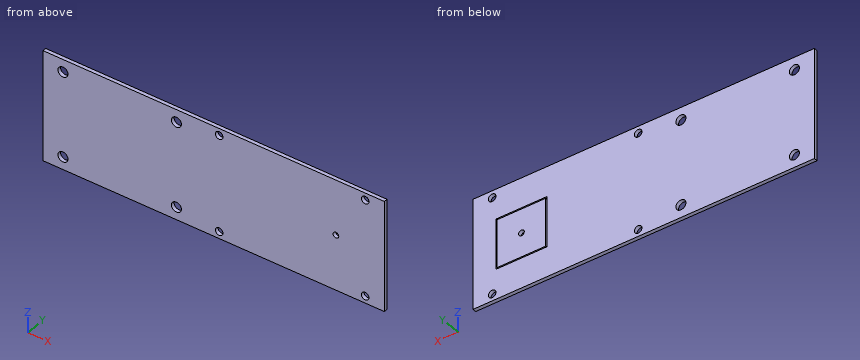
```python
from build123d import *

# Parameters (mm, degrees)
SKETCH1_W               = 141.05
SKETCH1_H               = 46
SKETCH1_R               = 2.075
SKETCH1_R_2             = 1.575
SKETCH1_R_3             = 1.185
BOSS_EXTRUDE1_DEPTH     = 1.5
SKETCH2_W               = 21
SKETCH2_H               = 21
SKETCH2_W_2             = 20
SKETCH2_H_2             = 20
CUT_EXTRUDE_THIN1_DEPTH = 0.75


with BuildPart() as part:
    # Sketch1 → Boss-Extrude1 (new body)
    with BuildSketch(Plane(origin=(0, 0, 0), x_dir=(1, 0, 0), z_dir=(0, 1, 0))):
        Rectangle(SKETCH1_W, SKETCH1_H)
        with Locations(Location((-62.28, -17.75, 0), (0, 0, 270))):
            Circle(SKETCH1_R, mode=Mode.SUBTRACT)
        with Locations(Location((-15.4, -17.75, 0), (0, 0, 270))):
            Circle(SKETCH1_R, mode=Mode.SUBTRACT)
        with Locations(Location((-15.4, 17.75, 0), (0, 0, 270))):
            Circle(SKETCH1_R, mode=Mode.SUBTRACT)
        with Locations(Location((-62.28, 17.75, 0), (0, 0, 270))):
            Circle(SKETCH1_R, mode=Mode.SUBTRACT)
        with Locations(Location((2.27, -20.09, 0), (0, 0, 270))):
            Circle(SKETCH1_R_2, mode=Mode.SUBTRACT)
        with Locations(Location((62.6, -20.09, 0), (0, 0, 270))):
            Circle(SKETCH1_R_2, mode=Mode.SUBTRACT)
        with Locations(Location((62.6, 20.09, 0), (0, 0, 270))):
            Circle(SKETCH1_R_2, mode=Mode.SUBTRACT)
        with Locations(Location((2.27, 20.09, 0), (0, 0, 270))):
            Circle(SKETCH1_R_2, mode=Mode.SUBTRACT)
        with Locations(Location((50.51, 0, 0), (0, 0, 270))):
            Circle(SKETCH1_R_3, mode=Mode.SUBTRACT)
    extrude(amount=BOSS_EXTRUDE1_DEPTH)

    # Sketch2 → Cut-Extrude-Thin1 (cut)
    with BuildSketch(Plane(origin=(0, 1.5, 0), x_dir=(1, 0, 0), z_dir=(0, 1, 0))):
        with Locations((50.51, 0)):
            Rectangle(SKETCH2_W, SKETCH2_H)
        with Locations((50.51, 0)):
            Rectangle(SKETCH2_W_2, SKETCH2_H_2, mode=Mode.SUBTRACT)
    extrude(amount=-CUT_EXTRUDE_THIN1_DEPTH, mode=Mode.SUBTRACT)


solid = part.part
```
Read the model definition and answer for the solid it produces. Units are mm, in the model's axes. Round coordinates to 2 decimals unless told otherwise and drop trailing zeros. Write each loop counter-clockwise with the first axis right and the second up, starting at its lowest first coordinate (ties: lowest second). Pieces come first, ordered by that corner, then holes. Notation, with made-up numbers: M 80.25,80 L 87.25,80 A25 ccw 87.25,103 Z; hole C -22,41 d5. An arc over 180 degrees is marked long. One line per item, written item: value.
Q1. Flat-ended cylindrical pins translate along their axes: pin 1 Ø6.5 at (x, z) = (-15.4, 17.75) entering from -Y; pin 2 Ø2.5 at (x, z) = (2.27, 20.09) entering from -Y. Find the tip coordinate at first contact, or state that the pin passes through.
Data:
pin 1: y = 0
pin 2: through
Q2. Find section B-B on x = 62.6. Write down the section's boundary in (y, z) (3 decimals).
Data:
outline: M 0,-23 L 1.5,-23 L 1.5,-21.665 L 0,-21.665 Z; M 0,-18.515 L 1.5,-18.515 L 1.5,18.515 L 0,18.515 Z; M 0,21.665 L 1.5,21.665 L 1.5,23 L 0,23 Z
Q3. Find section C-C on z = -17. Write down the section's boundary in (x, y) (3 decimals).
Data:
outline: M -70.525,0 L -64.215,0 L -64.215,1.5 L -70.525,1.5 Z; M -60.345,0 L -17.335,0 L -17.335,1.5 L -60.345,1.5 Z; M -13.465,0 L 70.525,0 L 70.525,1.5 L -13.465,1.5 Z
Q4. Straight lines are drawn through the part: line 1 (X direction, y = 0.9, z = -20.09) (3 decimals); line 2 (X direction, y = 0.8, z = 9) (3 decimals); line 3 (X direction, y = 0.95, z = 0) (3 decimals). For each, find the intervals that lie inside material, in ascending order. Write a range as [from, to].
Data:
line 1: [-70.525, 0.695], [3.845, 61.025], [64.175, 70.525]
line 2: [-70.525, 40.01], [40.51, 60.51], [61.01, 70.525]
line 3: [-70.525, 40.01], [40.51, 49.325], [51.695, 60.51], [61.01, 70.525]
Q5. Find section A-A on y = 1. Count the separate pieces of the cut face and the enclosed holes in it, plus the area to 3 significant figures.
Data:
separate pieces: 2
enclosed holes: 10
area: 6,360 mm2
